from build123d import *

# Parameters (mm, degrees)
SKETCH_1_W          = 14.5
SKETCH_1_H          = 13
EXTRUDE_1_DEPTH     = 5.5
SKETCH_2_W          = 5.703148186
SKETCH_2_H          = 13
EXTRUDE_2_DEPTH     = 1
SKETCH_3_W          = 12.6
SKETCH_3_H          = 5.1
CUT_EXTRUDE_1_DEPTH = 9.5
SKETCH_4_W          = 10
SKETCH_4_H          = 1.5
EXTRUDE_3_DEPTH     = 9.5


with BuildPart() as part:
    # 草图1 → 凸台-拉伸1 (new body)
    with BuildSketch(Plane(origin=(0, 0, 0), x_dir=(1, 0, 0), z_dir=(0, 1, 0))):
        with Locations((-1.331183612, -2.01138088)):
            Rectangle(SKETCH_1_W, SKETCH_1_H)
    extrude(amount=EXTRUDE_1_DEPTH)

    # 草图2 → 凸台-拉伸2 (add)
    with BuildSketch(Plane(origin=(0, 5.5, 0), x_dir=(1, 0, 0), z_dir=(0, 1, 0))):
        with Locations((-5.729609519, -2.01138088)):
            Rectangle(SKETCH_2_W, SKETCH_2_H)
    extrude(amount=EXTRUDE_2_DEPTH)

    # 草图3 → 切除-拉伸1 (cut)
    with BuildSketch(Plane(origin=(5.918816388, 0, 0), x_dir=(0, 0, -1), z_dir=(1, 0, 0))):
        with Locations((-2.01138088, 2.75)):
            Rectangle(SKETCH_3_W, SKETCH_3_H)
    extrude(amount=-CUT_EXTRUDE_1_DEPTH, mode=Mode.SUBTRACT)

    # 草图4 → 凸台-拉伸3 (add)
    with BuildSketch(Plane(origin=(-3.581183612, 0, 0), x_dir=(0, 0, -1), z_dir=(1, 0, 0))):
        with Locations((-2.01138088, 1.55)):
            Rectangle(SKETCH_4_W, SKETCH_4_H)
    extrude(amount=EXTRUDE_3_DEPTH)


solid = part.part
Read the model definition and answer for the solid it produces. Units are mm, in the model's axes. A direction names the side the tool comes from. Round coordinates to 2 decimals unless told otherwise and drop trailing zeros. Write each loop counter-clockwise with the first axis right and the second up, starting at its lowest first coordinate (ties: lowest second). Pieces come first, ordered by that corner, then holes.
1. Given pin 1 Ø0.8 at (y, z) = (6, 1) entering from +X; pin 2 Ø3 at (x, z) = (3.5, 2) entering from +Y; pin 3 Ø1.5 at (y, z) = (3.5, 5.5) entering from +X, each flat-ended and moving along its own axis, determine where each tip first touches the part or whether it passes through.
2. The part is cut by section C-C, the plane y = 1.25. Determine the outline of the cut face in (x, z), then the cut area to 3 significant figures.
3. Which of the six approach directions +Z, -Z, +X, -X, +Y, -Y give full straight-line access (tool end or side, diameter ignored) to faces 5 (the face through (1, 5.5, 2)), 6 (the face through (1, 3, 8.311)), 7 (the face through (-1, 3, 8.511))?
4. Straight lines are drawn through the part: L1, parallel to Y at x = 1.5, z = 4.5; L2, parallel to Z at x = -3.5, y = 2; L3, parallel to Z at x = -1.75, y = 5. For each, find the intervals that lie inside material, in ascending order.
5. The part is cut by section A-A, the plane x = 3.5. Determine the outline of the cut face in (y, z).
6. The part is cut by section D-D, the plane y = 4.75. Determine the outline of the cut face in (x, z).
7. Determine the mould class of faces 1 (the face through (-6, 6.5, 2)), 2 (the face through (1, 2.3, 2)), 3 (the face through (-8.581, 3, 2)), 4 (the face through (-1, 0, 2)) for opening direction Y: pulls with the +Y half, pulls with the -Y half, needs draft (parallel to the pull), parting line crosses it, or undercut.
8. The part is cut by section B-B, the plane z = -2.5. Determine the outline of the cut face in (x, y).
Values:
1. pin 1: stops at x = -2.88
1. pin 2: stops at y = 5.5
1. pin 3: stops at x = -3.58
2. outline: (-8.58, -4.49) - (5.92, -4.49) - (5.92, -4.29) - (-3.58, -4.29) - (-3.58, -2.99) - (5.92, -2.99) - (5.92, 7.01) - (-3.58, 7.01) - (-3.58, 8.31) - (5.92, 8.31) - (5.92, 8.51) - (-8.58, 8.51) - close
2. area: 164 mm2
3. face 5: +Z, -Z, +X, +Y
3. face 6: +X
3. face 7: +Z, +X, -X, +Y, -Y
4. L1: y = 0 to 0.2, 0.8 to 2.3, 5.3 to 5.5
4. L2: z = -4.49 to -4.29, -2.99 to 7.01, 8.31 to 8.51
4. L3: z = -4.49 to -4.29, 8.31 to 8.51
5. outline: (0, -4.49) - (5.5, -4.49) - (5.5, 8.51) - (0, 8.51) - close; (0.8, -2.99) - (2.3, -2.99) - (2.3, 7.01) - (0.8, 7.01) - close; hole (0.2, -4.29) - (5.3, -4.29) - (5.3, 8.31) - (0.2, 8.31) - close
6. outline: (-8.58, -4.49) - (5.92, -4.49) - (5.92, -4.29) - (-3.58, -4.29) - (-3.58, 8.31) - (5.92, 8.31) - (5.92, 8.51) - (-8.58, 8.51) - close
7. face 1: pulls with the +Y half
7. face 2: undercut
7. face 3: needs draft
7. face 4: pulls with the -Y half
8. outline: (-8.58, 0) - (5.92, 0) - (5.92, 0.2) - (-3.58, 0.2) - (-3.58, 0.8) - (5.92, 0.8) - (5.92, 2.3) - (-3.58, 2.3) - (-3.58, 5.3) - (5.92, 5.3) - (5.92, 5.5) - (-2.88, 5.5) - (-2.88, 6.5) - (-8.58, 6.5) - close
